```python
from build123d import *

# Parameters (mm, degrees)
SKETCH1_R           = 2.75
BOSS_EXTRUDE1_DEPTH = 5
SKETCH3_R           = 5.5
CUT_EXTRUDE2_DEPTH  = 4
SKETCH5_R           = 1.5
CUT_EXTRUDE3_DEPTH  = 7
SKETCH6_R           = 1.5
CUT_EXTRUDE4_DEPTH  = 7
CUT_EXTRUDE5_START  = -7
SKETCH7_R           = 1.5
CUT_EXTRUDE5_DEPTH  = 7
SKETCH8_R           = 1.5
CUT_EXTRUDE6_DEPTH  = 7


with BuildPart() as part:
    # Sketch1 → Boss-Extrude1 (new body)
    with BuildSketch(Plane.XY):
        Polygon((0, 42), (0, -20), (46, -20), (46, 42), (41, 42), (41, 62), (5, 62), (5, 42), align=None)
        with Locations((23, 42)):
            Circle(SKETCH1_R, mode=Mode.SUBTRACT)
        with Locations((23, 0)):
            Circle(SKETCH1_R, mode=Mode.SUBTRACT)
    extrude(amount=BOSS_EXTRUDE1_DEPTH)

    # Sketch3 → Cut-Extrude2 (cut)
    with BuildSketch(Plane.XY.offset(5)):
        with Locations((23, 42)):
            Circle(SKETCH3_R)
        with Locations((23, 0)):
            Circle(SKETCH3_R)
    extrude(amount=-CUT_EXTRUDE2_DEPTH, mode=Mode.SUBTRACT)

    # Sketch5 → Cut-Extrude3 (cut)
    with BuildSketch(Plane.XZ.offset(20)):
        with Locations(Location((5, 2.5, 0), (0, 0, 270))):
            Circle(SKETCH5_R)
        with Locations(Location((41, 2.5, 0), (0, 0, 270))):
            Circle(SKETCH5_R)
    extrude(amount=-CUT_EXTRUDE3_DEPTH, mode=Mode.SUBTRACT)

    # Sketch6 → Cut-Extrude4 (cut)
    with BuildSketch(Plane.ZY.offset(-5)):
        with Locations((2.5, 47)):
            Circle(SKETCH6_R)
        with Locations((2.5, 57)):
            Circle(SKETCH6_R)
    extrude(amount=-CUT_EXTRUDE4_DEPTH, mode=Mode.SUBTRACT)

    # Sketch7 → Cut-Extrude5 (cut)
    with BuildSketch(Plane(origin=(41, 0, 0), x_dir=(0, 0, -1), z_dir=(1, 0, 0)).offset(CUT_EXTRUDE5_START)):
        with Locations(Location((-2.5, 47, 0), (0, 0, 180))):
            Circle(SKETCH7_R)
        with Locations(Location((-2.5, 57, 0), (0, 0, 180))):
            Circle(SKETCH7_R)
    extrude(amount=CUT_EXTRUDE5_DEPTH, mode=Mode.SUBTRACT)

    # Sketch8 → Cut-Extrude6 (cut)
    with BuildSketch(Plane(origin=(0, 62, 0), x_dir=(1, 0, 0), z_dir=(0, 1, 0))):
        with Locations(Location((15, -2.5, 0), (0, 0, 270))):
            Circle(SKETCH8_R)
        with Locations(Location((31, -2.5, 0), (0, 0, 270))):
            Circle(SKETCH8_R)
    extrude(amount=-CUT_EXTRUDE6_DEPTH, mode=Mode.SUBTRACT)


solid = part.part
```
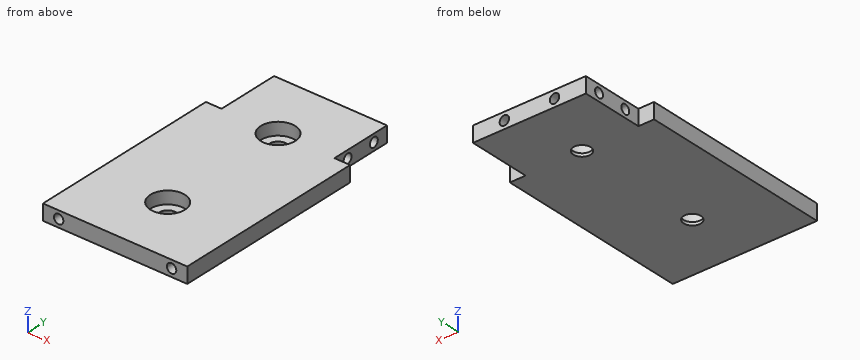
Work out the finished part from the listing and answer in its coordinate system (mm). Give positions to 0.01 mm unless a question says otherwise; leave off trailing zeros. Loops run counter-clockwise (first coordinate to the right, second up) from the corner with the lowest first, then second, coordinate; pieces in that order, holes last. Notation, with made-up numbers: (28.5, 50) - (40.5, 50) arc R14 ccw to (40.5, 68) - close; hole circle Ø7 at (-36, 83.25). An arc over 180 degrees is marked (long way). One line per question, with ' | ' between items.
(1) The part is cut by section B-B (x = 22). Write down the section's boundary in (y, z).
Recorded:
outline: (-20, 0) - (-2.56, 0) - (-2.56, 1) - (-5.41, 1) - (-5.41, 5) - (-20, 5) - close; (2.56, 0) - (39.44, 0) - (39.44, 1) - (36.59, 1) - (36.59, 5) - (5.41, 5) - (5.41, 1) - (2.56, 1) - close; (44.56, 0) - (62, 0) - (62, 5) - (47.41, 5) - (47.41, 1) - (44.56, 1) - close
(2) The part is cut by section D-D (x = 31). Write down the section's boundary in (y, z).
Recorded:
outline: (-20, 0) - (62, 0) - (62, 1) - (55, 1) - (55, 4) - (62, 4) - (62, 5) - (-20, 5) - close
(3) Each of these flat-tipped pins is pushed along its axis until it touches: pin 1 Ø0.9 at (y, z) = (57.5, 3) entering from +X; pin 2 Ø1.8 at (y, z) = (57, 2.5) entering from -X; pin 3 Ø9 at (x, y) = (23, 42) entering from +Z. Where does it stop, or does it pass through?
Recorded:
pin 1: stops at x = 34 | pin 2: stops at x = 12 | pin 3: stops at z = 1
(4) Straight lines are drawn through the part: probe 1 along Y at (x, z) = (36.75, 2.5); probe 2 along X at (y, z) = (-16.75, 2.5); probe 3 along Y at (x, z) = (23, 0.65). For each, find the intervals that lie inside material, in ascending order.
Recorded:
probe 1: y = -20 to 45.5, 48.5 to 55.5, 58.5 to 62 | probe 2: x = 0 to 3.5, 6.5 to 39.5, 42.5 to 46 | probe 3: y = -20 to -2.75, 2.75 to 39.25, 44.75 to 62
(5) The part is cut by section C-C (z = 2.5). Count the separate pieces of the cut face and the enclosed holes in it, then the cut area to 3 significant figures.
Recorded:
separate pieces: 1 | enclosed holes: 2 | area: 3,210 mm²
(6) The part is cut by section A-A (y = 0). Write down the section's boundary in (x, z).
Recorded:
outline: (0, 0) - (20.25, 0) - (20.25, 1) - (17.5, 1) - (17.5, 5) - (0, 5) - close; (25.75, 0) - (46, 0) - (46, 5) - (28.5, 5) - (28.5, 1) - (25.75, 1) - close
